```python
from build123d import *

# Parameters (mm, degrees)
SKETCH_1_R          = 11
EXTRUDE_1_DEPTH     = 8
SKETCH_2_W          = 30
SKETCH_2_H          = 8
SKETCH_2_R          = 3
EXTRUDE_2_DEPTH     = 3
FILLET_1_R          = 10
EXTRUDE_START       = 8
SKETCH_1_2_R        = 11
EXTRUDE_3_DEPTH     = 1
SKETCH_3_R          = 4
CUT_EXTRUDE_1_DEPTH = 31
SKETCH_4_R          = 6.25
CUT_EXTRUDE_2_DEPTH = 0.4


with BuildPart() as part:
    # 草圖1 → 填料-伸長1 (new body)
    with BuildSketch(Plane(origin=(0, 0, 0), x_dir=(1, 0, 0), z_dir=(0, 1, 0))):
        with BuildLine():
            Line((-15, 0), (-15, 30))
            Line((-15, 30), (15, 30))
            Line((15, 30), (15, 0))
            ThreePointArc((15, 0), (0, -15), (-15, 0))
        make_face()
        Circle(SKETCH_1_R, mode=Mode.SUBTRACT)
    extrude(amount=EXTRUDE_1_DEPTH)

    # 草圖2 → 填料-伸長2 (add)
    with BuildSketch(Plane(origin=(0, 0, -30), x_dir=(-1, 0, 0), z_dir=(0, 0, -1))):
        with Locations((0, 4)):
            Rectangle(SKETCH_2_W, SKETCH_2_H)
        with Locations((-10.5, 4)):
            Circle(SKETCH_2_R, mode=Mode.SUBTRACT)
        with Locations((10.5, 4)):
            Circle(SKETCH_2_R, mode=Mode.SUBTRACT)
        with BuildLine():
            Line((15, 32.5), (15, 8))
            Line((15, 8), (-15, 8))
            Line((-15, 8), (-15, 32.5))
            ThreePointArc((-15, 32.5), (-13.681980515, 35.681980515), (-10.5, 37))
            Line((-10.5, 37), (10.5, 37))
            ThreePointArc((10.5, 37), (13.681980515, 35.681980515), (15, 32.5))
        make_face()
        with Locations((10.5, 32.5)):
            Circle(SKETCH_2_R, mode=Mode.SUBTRACT)
        with Locations((-10.5, 32.5)):
            Circle(SKETCH_2_R, mode=Mode.SUBTRACT)
    extrude(amount=EXTRUDE_2_DEPTH)

    # 圓角1
    fillet_1_edges = [part.edges().sort_by_distance(p)[0] for p in [
        (0, 8, -30),
    ]]
    fillet(fillet_1_edges, radius=FILLET_1_R)

    # 草圖1<2> → 填料-伸長3 (add)
    with BuildSketch(Plane(origin=(0, 0, 0), x_dir=(1, 0, 0), z_dir=(0, 1, 0)).offset(EXTRUDE_START)):
        Circle(SKETCH_1_2_R)
    extrude(amount=-EXTRUDE_3_DEPTH)

    # 草圖3 → 除料-伸長1 (cut, through all)
    with BuildSketch(Plane(origin=(0, 7, 0), x_dir=(-1, 0, 0), z_dir=(0, -1, 0))):
        Circle(SKETCH_3_R)
    extrude(amount=-CUT_EXTRUDE_1_DEPTH, mode=Mode.SUBTRACT)

    # 草圖4 → 除料-伸長2 (cut)
    with BuildSketch(Plane(origin=(0, 7, 0), x_dir=(-1, 0, 0), z_dir=(0, -1, 0))):
        Circle(SKETCH_4_R)
    extrude(amount=-CUT_EXTRUDE_2_DEPTH, mode=Mode.SUBTRACT)


solid = part.part
```
Geometry: final body of the model. Coordinates: model frame, mm. A direction names the side the tool comes from. Give positions to 0.01 mm unless a question says otherwise; leave off trailing zeros. Loops run counter-clockwise (first coordinate to the right, second up) from the corner with the lowest first, then second, coordinate; pieces in that order, holes last. Notation, with made-up numbers: (5.5, 78) -> (34.5, 78) arc R20 ccw to (34.5, 115) -> close; hole circle Ø7 at (49, 3). An arc over 180 degrees is marked (long way). Return JSON: item names as keys, results as strings.
Item 1: Pin query (flat end, axial travel): P1, Ø1.5, axis at x = -11, y = 26.5, coming from the +Z side; P2, Ø10, axis at x = -1.5, z = -19, coming from the +Y side; P3, Ø10, axis at x = 0, z = 0, coming from the -Y side; P4, Ø5.5, axis at x = -10.5, y = 32.5, coming from the -Z side. Return the tip coordinate at first contact, or that it passes through.
Filled in:
{"P1": "z = -30", "P2": "y = 8.83", "P3": "y = 7.4", "P4": "through"}
Item 2: Section B-B, the plane y = 4. Output: boundary loops of the cut face in (x, z).
Filled in:
{"outline": "(-15, -33) -> (-13.5, -33) -> (-13.5, -30) -> (-7.5, -30) -> (-7.5, -33) -> (7.5, -33) -> (7.5, -30) -> (13.5, -30) -> (13.5, -33) -> (15, -33) -> (15, 0) arc R15 ccw to (-15, 0) -> close; hole circle Ø22 at (0, 0)"}
Item 3: Section D-D, the plane y = 25.5. Output: boundary loops of the cut face in (x, z).
Filled in:
{"outline": "(-15, -33) -> (15, -33) -> (15, -30) -> (-15, -30) -> close"}
Item 4: Section A-A, the plane x = 0. Output: boundary loops of the cut face in (y, z), plus the area to 3 significant figures.
Filled in:
{"outline": "(0, -33) -> (37, -33) -> (37, -30) -> (18, -30) arc R10 cw to (8, -20) -> (8, -4) -> (7.4, -4) -> (7.4, -6.25) -> (7, -6.25) -> (7, -11) -> (0, -11) -> close; (0, 11) -> (7, 11) -> (7, 6.25) -> (7.4, 6.25) -> (7.4, 4) -> (8, 4) -> (8, 15) -> (0, 15) -> close", "area": "329 mm^2"}
Item 5: Access query for faces 4 (the flat face through (0, 28, -30)), 5 (the cylindrical face through (-8.1, 2.2, -31.5)), 6 (the cylindrical face through (12.71, 34.53, -31.48)), 7 (the flat face through (-1.3, 7.4, 4.1)). Directions: +Z, -Z, +X, -X, +Y, -Y. A direction counts if a zero-diameter tool reaches every point of the face in a straight line with its end or side. Return the directions, or none.
Filled in:
{"face 4": "+Z, +X, -X, +Y", "face 5": "-Z", "face 6": "+Z, -Z", "face 7": "-Y"}
Item 6: Line query: line 1 (Y direction, x = 10.5, z = -30.9); line 2 (Z direction, x = 10, y = 35.5); line 3 (Z direction, x = 0, y = 2). Output: solid intervals per line, ascending.
Filled in:
{"line 1": "0 to 1, 7 to 29.5, 35.5 to 37", "line 2": "-33 to -30", "line 3": "-33 to -11, 11 to 15"}
Item 7: Section C-C, the plane z = -13. Output: boundary loops of the cut face in (x, y).
Filled in:
{"outline": "(-15, 0) -> (15, 0) -> (15, 8) -> (-15, 8) -> close"}
Item 8: Mould query, pull axis Z, two halves, no side actions, for faces 1 (the cylindrical face through (-5.96, 7.2, -1.88)), 2 (the cylindrical face through (12.9, 2.2, -31.5)), 3 (the flat face through (-11, 4, -30)). Classes: released by +Z, released by -Z, zero draft, split by the parting line, or undercut.
Filled in:
{"face 1": "undercut", "face 2": "zero draft", "face 3": "released by -Z"}
